Drawing for the job (mm, zero at the part's lowest x, y, z). A direction names the side the tool comes from. Coordinates: 2 decimals unless noted, no trailing zeros. Order: outer loops, then holes, each group sorted by start corner. A loop starts at its lowest first (then second) coordinate and runs counter-clockwise, first axis right, second up. Notation, with made-up numbers: (-22.75, 61) - (19.25, 61) arc R26 cw to (19.25, 93) - close; hole circle Ø8 at (64.25, -33.5). An arc over 180 degrees is marked (long way). Answer as CSV lines item,"result". Start each with the question number.
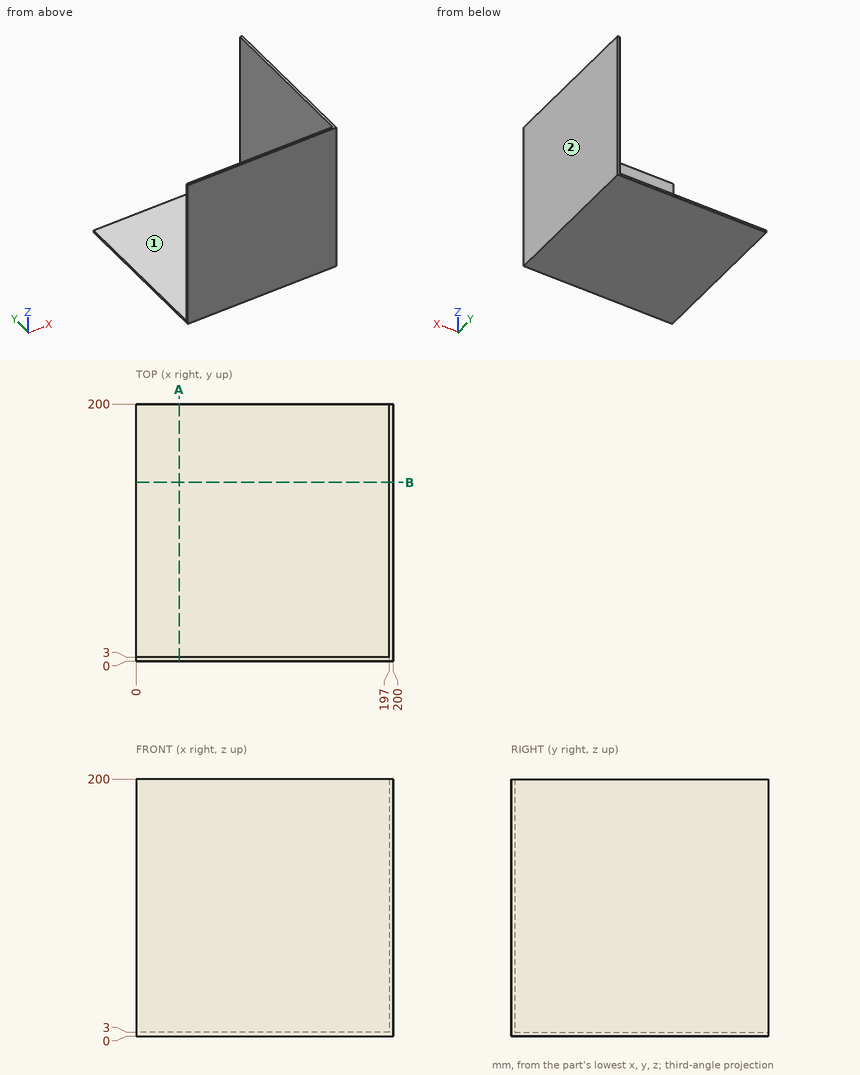
(1) Probe L1, parallel to Y at x = 74.5, z = 172.5; L2, parallel to X at y = 121, z = 189. List the from-to ranges inside material, lowest first. Write a range as [from, to].
(2) Band-saw the part on A-A on x = 33.5. List the corners of the cut face in (y, z), plus the area to 3 significant figures.
(3) Which spindle directions (+Z, -Z, +X, -X, +Y, -Y) get a long thin tool onto all of the face, cutting with end or side? Do the marked faces 1 and 2. Say none if no direction does.
(4) Drop flat-ended pins along their axis: pin 1 Ø5 at (x, y) = (164, 43.5) entering from -Z; pin 2 Ø2 at (y, z) = (36.5, 90.5) entering from -X; pin 3 Ø4 at (x, z) = (141.5, 54.5) entering from +Y; pin 4 Ø3 at (x, y) = (58, 104.5) entering from +Z. Give the stop position or say it passes through.
(5) Band-saw the part on B-B on y = 139. List the corners of the cut face in (x, z).
Filled in:
1,L1,"y = [0, 3]"
1,L2,"x = [197, 200]"
2,outline,"(0, 0) - (200, 0) - (200, 3) - (3, 3) - (3, 200) - (0, 200) - close"
2,area,"1,190 mm^2"
3,face 1,"+Z, -X, +Y"
3,face 2,"+Z, -Z, +X, +Y, -Y"
4,pin 1,"stops at z = 0"
4,pin 2,"stops at x = 197"
4,pin 3,"stops at y = 3"
4,pin 4,"stops at z = 3"
5,outline,"(0, 0) - (200, 0) - (200, 200) - (197, 200) - (197, 3) - (0, 3) - close"
